The listing builds one solid part. Answer for the finished solid, in the listing's coordinates (mm). A direction names the side the tool comes from. Round coordinates to 2 decimals unless told otherwise and drop trailing zeros. Write each loop counter-clockwise with the first axis right and the second up, starting at its lowest first coordinate (ties: lowest second). Pieces come first, ordered by that corner, then holes.
Item 1: Find section D-D on x = 0.5. Give the vertices of the cut face in (y, z).
Item 2: Find section A-A on x = -3.5. Give the vertices of the cut face in (y, z).
Item 3: For a pull along Y with two mould halves and no side action, classify faces 1 (the face through (-10.359, 7.797, 14.79)), 2 (the face through (0, -11, 15)), 3 (the face through (5, 10, 11.75)) as +Y half, -Y half, draft (parallel to the pull), parting line (faces both ways), or undercut.
Item 4: Each of these flat-tipped pins is pushed along its axis until it touches: pin 1 (1.5 mm diameter, centred on y = 3.5, z = 10, fed in from +X); pin 2 (6 mm diameter, centred on y = 3.5, z = 18, fed in from +X); pin 3 (8 mm diameter, centred on x = 0.5, z = 15, fed in from +Y); pin 4 (12 mm diameter, centred on x = -7.5, y = 4, fed in from +Z). Where does it stop, or does it pass through?
Item 5: Find the intervals of material crossed by probe 1 along Y at (x, z) = (1, 20.75); probe 2 along Z at (x, y) = (0.5, 10.05); probe 3 along X at (y, z) = (10.25, 15), in increasing order.
Item 6: Find section B-B on z = 15. Give the vertices of the cut face in (x, y), then the cut area to 3 significant figures.
Item 7: Find section C-C on z = 24.75. Give the vertices of the cut face in (x, y), then the cut area to 3 significant figures.
Item 8: A tool of negligible diameter and unlimited length cuts with its end or side. For faces 4 (the face through (9.5, 10, 15.1)), 5 (the face through (13.5, -10, 15)), 6 (the face through (5, 9, 11)), from which of +Z, -Z, +X, -X, +Y, -Y can it reach the whole face along a straight path? Write none if from no direction.
```python
from build123d import *

# Parameters (mm, degrees)
F1_DEPTH = 30
F3_DEPTH = 2


with BuildPart() as f1:
    # F0 (on Top) → F1 (new body)
    with BuildSketch(Plane.XY):
        with BuildLine():
            Line((-13.5, -11), (13.5, -11))
            Line((13.5, -11), (13.5, -9))
            Line((13.5, -9), (-11.5, -9))
            Line((-11.5, -9), (-11.5, 5))
            ThreePointArc((-11.5, 5), (-10.328427, 7.828427), (-7.5, 9))
            Line((-7.5, 9), (13.5, 9))
            Line((13.5, 9), (13.5, 11))
            Line((13.5, 11), (-13.5, 11))
            Line((-13.5, 11), (-13.5, -11))
        make_face()
    extrude(amount=F1_DEPTH)

    # F2 (on face) → F3 (cut, through all)
    with BuildSketch(Plane(origin=(0, 11, 0), x_dir=(-1, 0, 0), z_dir=(0, 1, 0))):
        with BuildLine():
            Line((-6.25, 11.75), (-4.299671, 11.75))
            Line((-4.299671, 11.75), (-0.5, 11.75))
            Line((-0.5, 11.75), (-0.5, 18.25))
            Line((-0.5, 18.25), (-4.299671, 18.25))
            Line((-4.299671, 18.25), (-6.25, 18.25))
            ThreePointArc((-6.25, 18.25), (-9.5, 15), (-6.25, 11.75))
        make_face()
        with BuildLine():
            Line((-0.5, 11.75), (-4.299671, 11.75))
            ThreePointArc((-4.299671, 11.75), (4.5, 15), (-4.299671, 18.25))
            Line((-4.299671, 18.25), (-0.5, 18.25))
            Line((-0.5, 18.25), (-0.5, 11.75))
        make_face()
    extrude(amount=-F3_DEPTH, mode=Mode.SUBTRACT)


solid = f1.part
```
Check values:
1. outline: (-11, 0) - (-9, 0) - (-9, 30) - (-11, 30) - close; (9, 0) - (11, 0) - (11, 10) - (9, 10) - close; (9, 20) - (11, 20) - (11, 30) - (9, 30) - close
2. outline: (-11, 0) - (-9, 0) - (-9, 30) - (-11, 30) - close; (9, 0) - (11, 0) - (11, 12) - (9, 12) - close; (9, 18) - (11, 18) - (11, 30) - (9, 30) - close
3. face 1: undercut
3. face 2: -Y half
3. face 3: draft
4. pin 1: stops at x = -11.5
4. pin 2: stops at x = -11.21
4. pin 3: stops at y = -9
4. pin 4: stops at z = 30
5. probe 1: y = -11 to -9, 9 to 11
5. probe 2: z = 0 to 10, 20 to 30
5. probe 3: x = -13.5 to -4.5, 9.5 to 13.5
6. outline: (-13.5, -11) - (13.5, -11) - (13.5, -9) - (-11.5, -9) - (-11.5, 5) arc R4 cw to (-7.5, 9) - (-4.5, 9) - (-4.5, 11) - (-13.5, 11) - close; (9.5, 9) - (13.5, 9) - (13.5, 11) - (9.5, 11) - close
6. area: 119 mm2
7. outline: (-13.5, -11) - (13.5, -11) - (13.5, -9) - (-11.5, -9) - (-11.5, 5) arc R4 cw to (-7.5, 9) - (13.5, 9) - (13.5, 11) - (-13.5, 11) - close
7. area: 147 mm2
8. face 4: +Y
8. face 5: +Z, -Z, +X, +Y, -Y
8. face 6: +Z, -Z, +X
